```python
from build123d import *

# Parameters (mm, degrees)
SKETCH1_R           = 4.525
BOSS_EXTRUDE1_DEPTH = 4
SKETCH2_W           = 29.05
SKETCH2_H           = 15
BOSS_EXTRUDE2_DEPTH = 3
SKETCH3_R           = 1.8
CUT_EXTRUDE1_DEPTH  = 37.906160055
FILLET1_R           = 3
FILLET2_R           = 1.5


with BuildPart() as part:
    # Sketch1 → Boss-Extrude1 (new body)
    with BuildSketch(Plane(origin=(0, 0, 0), x_dir=(1, 0, 0), z_dir=(0, 1, 0))):
        with BuildLine():
            Line((-14.525, 20.57), (-14.525, 0))
            Line((-14.525, 0), (14.525, 0))
            Line((14.525, 0), (14.525, 20.57))
            ThreePointArc((14.525, 20.57), (0, 35.095), (-14.525, 20.57))
        make_face()
        with Locations(Location((0, 20.57, 0), (0, 0, 270))):
            Circle(SKETCH1_R, mode=Mode.SUBTRACT)
    extrude(amount=BOSS_EXTRUDE1_DEPTH)

    # Sketch2 → Boss-Extrude2 (add)
    with BuildSketch(Plane.XY):
        with Locations((0, -3.5)):
            Rectangle(SKETCH2_W, SKETCH2_H)
    extrude(amount=-BOSS_EXTRUDE2_DEPTH)

    # Sketch3 → Cut-Extrude1 (cut, through all)
    with BuildSketch(Plane(origin=(0, 0, -3), x_dir=(-1, 0, 0), z_dir=(0, 0, -1))):
        with Locations((-7.2625, -5.5)):
            Circle(SKETCH3_R)
        with Locations(Location((7.2625, -5.5, 0), (0, 0, 180))):
            Circle(SKETCH3_R)
    extrude(amount=-CUT_EXTRUDE1_DEPTH, mode=Mode.SUBTRACT)

    # Fillet1
    fillet1_edges = [part.edges().sort_by_distance(p)[0] for p in [
        (-14.525, -11, -1.5),
        (0, 0, -3),
        (14.525, -11, -1.5),
    ]]
    fillet(fillet1_edges, radius=FILLET1_R)

    # Fillet2
    fillet2_edges = [part.edges().sort_by_distance(p)[0] for p in [
        (0, 0, -25.095),
        (0, 4, -25.095),
    ]]
    fillet(fillet2_edges, radius=FILLET2_R)


solid = part.part
```
The listing builds one solid part. Answer for the finished solid, in the listing's coordinates (mm). A direction names the side the tool comes from. Coordinates: 2 decimals unless noted, no trailing zeros. Loops run counter-clockwise (first coordinate to the right, second up) from the corner with the lowest first, then second, coordinate; pieces in that order, holes last. Notation, with made-up numbers: (78, 1.5) -> (114, 1.5) arc R18 ccw to (114, 31.5) -> close; hole circle Ø9 at (67, 76). An arc over 180 degrees is marked (long way). Use one line per item in the form item = value. Start each with the question number.
Item 1: The mould has two halves that part along Y. Classify faces 3 (the face through (-6.432, -3.903, -1.521)), 4 (the face through (0, -7, -3)), 5 (the face through (5.546, -4.959, -1.521)), 6 (the face through (0, -11, -1)): released by +Y, released by -Y, zero draft, split by the parting line, or undercut.
Item 2: The part is cut by section C-C on z = -11.5. Determine the outline of the cut face in (x, y) (3 decimals).
Item 3: Flat-ended cylindrical pins translate along their axes: pin 1 Ø4 at (x, y) = (1.5, -8.5) entering from -Z; pin 2 Ø2 at (x, y) = (10.5, -4) entering from +Z. Find the tip coordinate at first contact, or state that the pin passes through.
Item 4: The part is cut by section B-B on y = -5.5. Determine the outline of the cut face in (x, z) (1 decimal), then the cut area to 4 significant figures.
Item 5: A tool of negligible diameter and unlimited length cuts with its end or side. For faces 1 (the face through (-14.525, 1, -8)), 2 (the face through (0, 0, -14)), from which of +Z, -Z, +X, -X, +Y, -Y can it reach the whole face along a straight path? Write none if from no direction.
Item 6: Consider L1, parallel to X at y = -5, z = -2.5 (3 decimals); L2, parallel to Y at x = 3, z = -30; L3, parallel to Z at x = -3.75, y = -9. Determine where each line is inside the solid, lowest interval first. Write a range as [from, to].
Item 7: The part is cut by section A-A on x = 0. Determine the outline of the cut face in (y, z) (3 decimals), then the cut area to 3 significant figures.
Item 8: The part is cut by section D-D on y = -9.75. Determine the outline of the cut face in (x, z).
Answer key:
q1.face_3 = undercut
q1.face_4 = zero draft
q1.face_5 = undercut
q1.face_6 = released by -Y
q2.outline = (-14.525, 0) -> (14.525, 0) -> (14.525, 4) -> (-14.525, 4) -> close
q3.pin_1 = -3
q3.pin_2 = 0
q4.outline = (-14.5, -3) -> (-9.1, -3) -> (-9.1, 0) -> (-14.5, 0) -> close; (-5.5, -3) -> (5.5, -3) -> (5.5, 0) -> (-5.5, 0) -> close; (9.1, -3) -> (14.5, -3) -> (14.5, 0) -> (9.1, 0) -> close
q4.area = 65.55 mm2
q5.face_1 = +Z, -Z, -X, +Y, -Y
q5.face_2 = -Z, +X, -X, -Y
q6.L1 = [-14.525, -8.992], [-5.533, 5.533], [8.992, 14.525]
q6.L2 = [0, 4]
q6.L3 = [-3, 0]
q7.outline = (-11, -3) -> (-3, -3) arc R3 cw to (0, -6) -> (0, -14.545) arc R1.5 ccw to (1.5, -16.045) -> (2.5, -16.045) arc R1.5 ccw to (4, -14.545) -> (4, 0) -> (-11, 0) -> close; (0, -35.095) -> (4, -35.095) -> (4, -26.595) arc R1.5 ccw to (2.5, -25.095) -> (1.5, -25.095) arc R1.5 ccw to (0, -26.595) -> close
q7.area = 137 mm2
q8.outline = (-13.96, -3) -> (13.96, -3) -> (13.96, 0) -> (-13.96, 0) -> close
